Read the model definition and answer for the solid it produces. Units are mm, in the model's axes. Face numbers are marked on the shaded views. A direction names the side the tool comes from. Coordinates: 2 decimals unless noted, no trailing zeros.
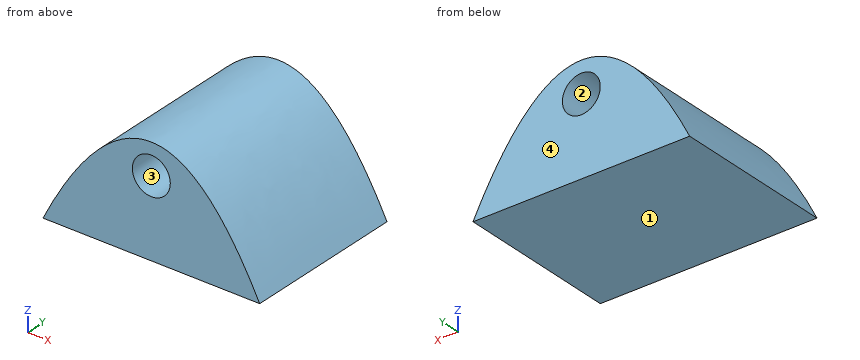
from build123d import *

# Parameters (mm, degrees)
BOSS_EXTRUDE1_DEPTH     = 300
SKETCH3_R               = 15.5
CUT_EXTRUDE1_DEPTH      = 23
CUT_EXTRUDE1_DEPTH_BACK = 23
SKETCH4_R               = 35
CUT_EXTRUDE3_DEPTH      = 300


with BuildPart() as part:
    # Sketch1 → Boss-Extrude1 (new body)
    with BuildSketch(Plane(origin=(0, 0, 0), x_dir=(1, 0, 0), z_dir=(0, 1, 0))):
        with BuildLine():
            Line((-200, 1e-09), (200, 1e-09))
            add(Edge.make_bspline(
                [(-200, 1e-09), (0, -400.000000001), (200, 1e-09)],
                knots=[0.056028396, 0.056028396, 0.056028396, 0.943971604, 0.943971604, 0.943971604], degree=2))
        make_face()
    extrude(amount=BOSS_EXTRUDE1_DEPTH)

    # Sketch3 → Cut-Extrude1 (cut, two sides)
    with BuildSketch(Plane(origin=(0, 150, 0), x_dir=(1, 0, 0), z_dir=(0, 1, 0))) as cut_extrude1_sk:
        with Locations((0, -142.999999999)):
            Circle(SKETCH3_R)
    extrude(amount=CUT_EXTRUDE1_DEPTH, mode=Mode.SUBTRACT)
    extrude(cut_extrude1_sk.sketch, amount=-CUT_EXTRUDE1_DEPTH_BACK, mode=Mode.SUBTRACT)

    # Sketch4 → Cut-Extrude3 (cut)
    with BuildSketch(Plane(origin=(0, 173, 0), x_dir=(1, 0, 0), z_dir=(0, 1, 0))):
        with Locations((0, -142.999999999)):
            Circle(SKETCH4_R)
    cut_extrude3 = extrude(amount=CUT_EXTRUDE3_DEPTH, mode=Mode.SUBTRACT)

    # Mirror1: Cut-Extrude3 across plane
    add(cut_extrude3.mirror(Plane.ZX.offset(150)), mode=Mode.SUBTRACT)


solid = part.part
Q1. Straight lines are drawn through the part: probe 1 along Z at (x, y) = (0, 33); probe 2 along Z at (x, y) = (0, 145); probe 3 along Y at (x, z) = (-5, 112.5). For each, find the intervals that lie inside material, in ascending order.
Findings below:
probe 1: z = 0 to 108, 178 to 200
probe 2: z = 0 to 127.5, 158.5 to 200
probe 3: y = 127 to 173
Q2. Determine the mould class of the marked faces 1 and 2 for opening direction X: +X half, -X half, draft (parallel to the pull), parting line (faces both ways), or undercut.
Findings below:
face 1: draft
face 2: undercut
Q3. Which of the six approach directions +Z, -Z, +X, -X, +Y, -Y give full straight-line access (tool end or side, diameter ignored) to the marked faces 3 and 4?
Findings below:
face 3: -Y
face 4: +Z, -Z, +X, -X, +Y
Q4. Flat-ended cylindrical pins translate along their axes: pin 1 Ø8 at (y, z) = (257, 165) entering from -X; pin 2 Ø2 at (x, z) = (17, 143) entering from +Y; pin 3 Ø18.5 at (x, z) = (0, 143) entering from -Y; pin 4 Ø8 at (y, z) = (162.5, 116.5) entering from -X. Find the tip coordinate at first contact, or state that the pin passes through.
Findings below:
pin 1: stops at x = -88.32
pin 2: stops at y = 173
pin 3: passes through
pin 4: stops at x = -132.29
